The model under review builds one solid part; all positions refer to its coordinate system, in mm. A direction names the side the tool comes from. Coordinates: 2 decimals unless noted, no trailing zeros. Order: outer loops, then holes, each group sorted by start corner. A loop starts at its lowest first (then second) coordinate and runs counter-clockwise, first axis right, second up. Notation, with made-up numbers: (67, -30) -> (103, -30) arc R12 ccw to (103, -25) -> close; hole circle Ø9 at (14, 62.5). An arc over 180 degrees is marked (long way). Use one line per item in the form item = value.
from build123d import *

# Parameters (mm, degrees)
AUFSATZ_LINEAR_AUSTRAGEN1_DEPTH  = 15
SCHNITT_LINEAR_AUSTRAGEN5_DEPTH  = 20.5
SCHNITT_LINEAR_AUSTRAGEN5_DRAFT  = -4
AUFSATZ_LINEAR_AUSTRAGEN4_DEPTH  = 2.5
AUFSATZ_LINEAR_AUSTRAGEN5_DEPTH  = 20.5
VERRUNDUNG1_R                    = 8
VERRUNDUNG2_R                    = 6
VERRUNDUNG3_R                    = 1
F_3_8_3_8_DURCHMESSER_BOHRUNG1_D = 3.8


with BuildPart() as part:
    # Skizze1 → Aufsatz-Linear austragen1 (new body)
    with BuildSketch(Plane.XY):
        Polygon((22.25, -56.552393395), (22.25, -2.472222222), (45, -2.472222222), (45, 2.472222222), (-45, 2.472222222), (-45, -2.472222222), (-22.25, -2.472222222), (-22.25, -56.552393395), (0, -59.024615617), align=None)
    extrude(amount=-AUFSATZ_LINEAR_AUSTRAGEN1_DEPTH)


with BuildPart() as schnitt_linear_austragen5_tool:
    # Skizze4 → Schnitt-Linear austragen5 (with draft: the straight prism first)
    with BuildSketch(Plane(origin=(0, 0, -15), x_dir=(-1, 0, 0), z_dir=(0, 0, -1))):
        with BuildLine():
            ThreePointArc((12.810057025, -3.435647478), (0, -2.7261607), (-12.810057025, -3.435647478))
            Line((-12.810057025, -3.435647478), (-20.25, -4.262307808))
            Line((-20.25, -4.262307808), (-20.25, -54.762307808))
            Line((-20.25, -54.762307808), (-12.810057025, -55.588968139))
            ThreePointArc((-12.810057025, -55.588968139), (0, -56.298454917), (12.810057025, -55.588968139))
            Line((12.810057025, -55.588968139), (20.25, -54.762307808))
            Line((20.25, -54.762307808), (20.25, -4.262307808))
            Line((20.25, -4.262307808), (12.810057025, -3.435647478))
        make_face()
    extrude(amount=-SCHNITT_LINEAR_AUSTRAGEN5_DEPTH)
    # Schnitt-Linear austragen5: the draft: its side faces are tilted about the plane it starts from
    schnitt_linear_austragen5_sides = [schnitt_linear_austragen5_tool.faces().sort_by_distance(p)[0] for p in [
        (0, -2.7261607, -4.75),
        (16.530028512, -3.848977643, -4.75),
        (20.25, -29.512307808, -4.75),
        (16.530028512, -55.175637974, -4.75),
        (0, -56.298454917, -4.75),
        (-16.530028512, -55.175637974, -4.75),
        (-20.25, -29.512307808, -4.75),
        (-16.530028512, -3.848977643, -4.75),
    ]]
    draft(schnitt_linear_austragen5_sides, Plane(origin=(0, 0, -15), x_dir=(-1, 0, 0), z_dir=(0, 0, -1)), SCHNITT_LINEAR_AUSTRAGEN5_DRAFT)


with BuildPart() as part_1:
    add(part.part)

    # Schnitt-Linear austragen5: cut by schnitt_linear_austragen5_tool
    add(schnitt_linear_austragen5_tool.part, mode=Mode.SUBTRACT)

    # Skizze1_6 → Aufsatz-Linear austragen4 (add)
    # profile 1 of 4: a face of its own
    with BuildSketch(Plane.XY):
        Polygon((22.25, -2.472222222), (0, 0), (-22.25, -2.472222222), align=None)
    # profile 2 of 4: a face of its own
    with BuildSketch(Plane.XY):
        Polygon((-22.25, -2.472222222), (0, 0), (22.25, -2.472222222), (45, -2.472222222), (45, 2.472222222), (-45, 2.472222222), (-45, -2.472222222), align=None)
    # profile 3 of 4: a face of its own
    with BuildSketch(Plane.XY):
        Polygon((22.25, -56.552393395), (22.25, -2.472222222), (-22.25, -2.472222222), (-22.25, -56.552393395), (0, -59.024615617), align=None)
        with BuildLine():
            ThreePointArc((-12.810057025, -3.435647478), (0, -2.7261607), (12.810057025, -3.435647478))
            Line((12.810057025, -3.435647478), (20.25, -4.262307808))
            Line((20.25, -4.262307808), (20.25, -54.762307808))
            Line((20.25, -54.762307808), (12.810057025, -55.588968139))
            ThreePointArc((12.810057025, -55.588968139), (0, -56.298454917), (-12.810057025, -55.588968139))
            Line((-12.810057025, -55.588968139), (-20.25, -54.762307808))
            Line((-20.25, -54.762307808), (-20.25, -4.262307808))
            Line((-20.25, -4.262307808), (-12.810057025, -3.435647478))
        make_face(mode=Mode.SUBTRACT)
    # profile 4 of 4: a face of its own
    with BuildSketch(Plane.XY):
        with BuildLine():
            ThreePointArc((12.810057025, -55.588968139), (0, -56.298454917), (-12.810057025, -55.588968139))
            Line((-12.810057025, -55.588968139), (-20.25, -54.762307808))
            Line((-20.25, -54.762307808), (-20.25, -4.262307808))
            Line((-20.25, -4.262307808), (-12.810057025, -3.435647478))
            ThreePointArc((-12.810057025, -3.435647478), (0, -2.7261607), (12.810057025, -3.435647478))
            Line((12.810057025, -3.435647478), (20.25, -4.262307808))
            Line((20.25, -4.262307808), (20.25, -54.762307808))
            Line((20.25, -54.762307808), (12.810057025, -55.588968139))
        make_face()
    extrude(amount=AUFSATZ_LINEAR_AUSTRAGEN4_DEPTH)

    # Skizze1_7 → Aufsatz-Linear austragen5 (add)
    with BuildSketch(Plane.XY):
        Polygon((-22.25, -2.472222222), (0, 0), (22.25, -2.472222222), (45, -2.472222222), (45, 2.472222222), (-45, 2.472222222), (-45, -2.472222222), align=None)
        Polygon((22.25, -2.472222222), (0, 0), (-22.25, -2.472222222), align=None)
    extrude(amount=AUFSATZ_LINEAR_AUSTRAGEN5_DEPTH)

    # Verrundung1
    verrundung1_edges = [part_1.edges().sort_by_distance(p)[0] for p in [
        (0, -2.472222222, 2.5),
        (22.25, -2.472222222, -6.25),
        (-22.25, -2.472222222, -6.25),
    ]]
    fillet(verrundung1_edges, radius=VERRUNDUNG1_R)

    # Verrundung2
    verrundung2_edges = [part_1.edges().sort_by_distance(p)[0] for p in [
        (-45, 0, 20.5),
        (45, 0, 20.5),
        (-45, 0, -15),
        (45, 0, -15),
    ]]
    fillet(verrundung2_edges, radius=VERRUNDUNG2_R)

    # Verrundung3
    verrundung3_edges = [part_1.edges().sort_by_distance(p)[0] for p in [
        (-11.125, -57.788504506, 2.5),
        (11.125, -57.788504506, 2.5),
        (22.25, -33.512307808, 2.5),
        (22.25, -33.512307808, -15),
        (34.625, -2.472222222, -15),
        (-11.125, -57.788504506, -15),
        (-22.25, -33.512307808, 2.5),
        (-22.25, -33.512307808, -15),
        (24.593145751, -4.815367973, -15),
        (-24.593145751, -4.815367973, -15),
        (-25.081608741, -4.365854088, 5.331608741),
        (25.081608741, -4.365854088, 5.331608741),
        (45, -2.472222222, 2.75),
        (-34.625, -2.472222222, -15),
        (0, -2.472222222, 20.5),
        (-45, -2.472222222, 2.75),
        (-43.242640687, -2.472222222, 18.742640687),
        (43.242640687, -2.472222222, 18.742640687),
        (-43.242640687, -2.472222222, -13.242640687),
        (43.242640687, -2.472222222, -13.242640687),
        (11.125, -57.788504506, -15),
        (22.25, -56.552393395, -6.25),
        (-22.25, -56.552393395, -6.25),
    ]]
    fillet(verrundung3_edges, radius=VERRUNDUNG3_R)

    # 3.8 _3.8_ Durchmesser Bohrung1 (through all)
    with Locations(Plane(origin=(-37, -2.472222222, 0), x_dir=(0, 0, -1), z_dir=(0, -1, 0))):
        with Locations((0, 0), (0, 74)):
            Hole(F_3_8_3_8_DURCHMESSER_BOHRUNG1_D / 2)


solid = part_1.part
Item 1: We need section C-C (z = -3). Write out the cut boundary in (x, y).
Results found:
outline = (-45, -1.47) arc R1 ccw to (-44, -2.47) -> (-30.25, -2.47) arc R8 cw to (-22.25, -10.47) -> (-22.25, -55.66) arc R1 ccw to (-21.36, -56.65) -> (0, -59.02) -> (21.36, -56.65) arc R1 ccw to (22.25, -55.66) -> (22.25, -10.47) arc R8 cw to (30.25, -2.47) -> (44, -2.47) arc R1 ccw to (45, -1.47) -> (45, 2.47) -> (-45, 2.47) -> close; hole (-19.41, -54.01) -> (-12.72, -54.75) arc R115.16 ccw to (12.72, -54.75) -> (19.41, -54.01) -> (19.41, -5.01) -> (12.72, -4.27) arc R115.16 ccw to (-12.72, -4.27) -> (-19.41, -5.01) -> close
Item 2: To check wall thickness, follow L1, parallel to X at y = -1.35, z = 0; L2, parallel to Y at x = 37, z = -6; L3, parallel to X at y = -23, z = -2.5. State the ranges of each line that lie inside material, in increasing order. Write a range as from..to.
Results found:
L1 = -45..-38.9, -35.1..35.1, 38.9..45
L2 = -2.47..2.47
L3 = -22.25..-19.38, 19.38..22.25
Item 3: We need section B-B (y = -18.5). Write out the cut boundary in (x, z), plus the area to 3 significant figures.
Results found:
outline = (-22.25, -14) arc R1 ccw to (-21.25, -15) -> (-20.25, -15) -> (-19.2, 0) -> (19.2, 0) -> (20.25, -15) -> (21.25, -15) arc R1 ccw to (22.25, -14) -> (22.25, 1.5) arc R1 ccw to (21.25, 2.5) -> (-21.25, 2.5) arc R1 ccw to (-22.25, 1.5) -> close
area = 186 mm²
Item 4: Clearance check with flat-ended pins moving along their axes: pin 1 (1 mm diameter, centred on y = -32.5, z = -2, fed in from +X); pin 2 (5 mm diameter, centred on x = 4.5, y = -10.5, fed in from +Z); pin 3 (4.5 mm diameter, centred on x = 37, z = 0, fed in from -Y). State where each tip first meets the part, or that it passes through.
Results found:
pin_1 = 22.25
pin_2 = 2.89
pin_3 = -2.47
Item 5: Tool access review of faces 4 (the face through (-45, 1, 3)), 5 (the face through (16.421, -4.357, -7.605)), 6 (the face through (-1, -2.472, 14)): name each direction out of +Z, -Z, +X, -X, +Y, -Y from which nothing blocks a thin tool from reaching the whole face with its end or side.
Results found:
face_4 = +Z, -Z, -X, +Y, -Y
face_5 = -Z
face_6 = +Z, -Y
Item 6: Draft analysis for pull direction Y (two halves, no side actions). For faces 1 (the face through (0.18, -55.78, -7.6)), 2 (the face through (-10.5, -57.56, -14.71)), 3 (the face through (-6, -1, -15)), state which applies: released by +Y, released by -Y, zero draft, split by the parting line, or undercut.
Results found:
face_1 = undercut
face_2 = released by -Y
face_3 = zero draft
Item 7: We need section A-A (x = 37). Write out the cut boundary in (y, z), plus the area to 3 significant figures.
Results found:
outline = (-2.47, -14) arc R1 ccw to (-1.47, -15) -> (2.47, -15) -> (2.47, -1.9) -> (-2.47, -1.9) -> close; (-2.47, 1.9) -> (2.47, 1.9) -> (2.47, 20.5) -> (-1.47, 20.5) arc R1 ccw to (-2.47, 19.5) -> close
area = 156 mm²
